from build123d import *

# Parameters (mm, degrees)
F0_W      = 58
F0_H      = 54
F1_DEPTH  = 10
F3_DEPTH  = 10
F5_DEPTH  = 50
F4_R      = 6
F4_W      = 10
F4_H      = 44
F7_DEPTH  = 50
F9_DEPTH  = 62.001
F10_DEPTH = 60.001
F11_DEPTH = 10.001


with BuildPart() as f1:
    # F0 (on Top) → F1 (new body)
    with BuildSketch(Plane.XY):
        Rectangle(F0_W, F0_H)
        Polygon((-29, -27), (-29, 27), (-81, 27), (-81, 7), align=None)
    extrude(amount=F1_DEPTH)

    # F2 (on face) → F3 (join)
    with BuildSketch(Plane(origin=(0, 27, 0), x_dir=(-1, 0, 0), z_dir=(0, 1, 0))):
        Polygon((19, 60), (-29, 10), (19, 10), align=None)
    extrude(amount=-F3_DEPTH)

    # F4 (on face) → F5 (join)
    with BuildSketch(Plane.XY.offset(10)):
        Polygon((-81, 27), (-81, 17), (-29, 17), (-19, 17), (-19, 27), align=None)
    extrude(amount=F5_DEPTH)

    # F4 (on face) → F7 (join)
    with BuildSketch(Plane.XY.offset(10)):
        with Locations((17, -5)):
            Circle(F4_R)
        with Locations((-5, -5)):
            Circle(F4_R)
        with Locations((-24, -5)):
            Rectangle(F4_W, F4_H)
    extrude(amount=F7_DEPTH)

    # F8 (on face) → F9 (cut, through all)
    with BuildSketch(Plane.YZ.offset(-19)):
        Polygon((-27, 60), (-27, 10), (17, 60), align=None)
    extrude(amount=-F9_DEPTH, mode=Mode.SUBTRACT)

    # F10 (cut, through all): faces of the model
    f10_faces = [f1.faces().sort_by_distance(p)[0] for p in [
        (-5, -5, 60),
        (17, -5, 60),
    ]]
    extrude(f10_faces, amount=-F10_DEPTH, mode=Mode.SUBTRACT)

    # F6 (on face) → F11 (cut, through all)
    with BuildSketch(Plane.XZ.offset(-17)):
        with BuildLine():
            ThreePointArc((-56.470110421, 44), (-59.8754155453, 47.4053051244), (-63.2807206697, 44))
            Line((-63.2807206697, 44), (-63.2807206697, 24))
            ThreePointArc((-63.2807206697, 24), (-59.8754155453, 20.5946948756), (-56.470110421, 24))
            Line((-56.470110421, 24), (-56.470110421, 44))
        make_face()
        with BuildLine():
            ThreePointArc((-34.5057800598, 44), (-37.8754155453, 47.3696354855), (-41.2450510308, 44))
            Line((-41.2450510308, 44), (-41.2450510308, 24))
            ThreePointArc((-41.2450510308, 24), (-37.8754155453, 20.6303645145), (-34.5057800598, 24))
            Line((-34.5057800598, 24), (-34.5057800598, 44))
        make_face()
    extrude(amount=-F11_DEPTH, mode=Mode.SUBTRACT)


solid = f1.part
Could you check a few things on this model? Use its own coordinates, in mm. A direction names the side the tool comes from. Round coordinates to 2 decimals unless told otherwise and drop trailing zeros. Loops run counter-clockwise (first coordinate to the right, second up) from the corner with the lowest first, then second, coordinate; pieces in that order, holes last. Notation, with made-up numbers: (7, -24.75) - (54, -24.75) arc R9 ccw to (54, -16.75) - close; hole circle Ø7 at (69.25, 68). An arc over 180 degrees is marked (long way). Write item = value, one per line.
1) I need wall thicknesses on line 1 along Z through (x, y) = (5, -7); line 2 along X through (y, z) = (9.5, 21.5); line 3 along Y through (x, z) = (-51.5, 37.5). Which ranges of each line are inside material? Lowest first, please. Write a range as from..to.
Computed:
line_1 = 0..10
line_2 = -29..-19
line_3 = 17..27
2) Imagine slicing it at C-C (z = 55). Please give me the cut outline in (x, y).
Computed:
outline = (-81, 17) - (-29, 17) - (-29, 12.6) - (-19, 12.6) - (-19, 17) - (-14.2, 17) - (-14.2, 27) - (-81, 27) - close
3) Imagine slicing it at D-D (y = 19). Please give me the cut outline in (x, z).
Computed:
outline = (-81, 0) - (29, 0) - (29, 10) - (-19, 60) - (-81, 60) - close; hole (-63.28, 24) arc R3.41 ccw to (-56.47, 24) - (-56.47, 44) arc R3.41 ccw to (-63.28, 44) - close; hole (-41.25, 24) arc R3.37 ccw to (-34.51, 24) - (-34.51, 44) arc R3.37 ccw to (-41.25, 44) - close
4) If we mould it in two halves opening along Z, with no side actions, what happens to faces 6 (the flat face through (-24, -5, 35)), 7 (the cylindrical face through (-59.95, 21.93, 20.596)), 8 (the flat face through (-55, 17, 35))? For each: pulls with the +Z half, pulls with the -Z half, needs draft (parallel to the pull), parting line crosses it, or undercut.
Computed:
face_6 = pulls with the +Z half
face_7 = undercut
face_8 = needs draft
5) Imagine slicing it at A-A (x = 17). Please give me the cut outline in (y, z), and give its area (3 significant figures).
Computed:
outline = (-27, 0) - (-11, 0) - (-11, 10) - (-27, 10) - close; (1, 0) - (27, 0) - (27, 22.5) - (17, 22.5) - (17, 10) - (1, 10) - close
area = 545 mm2
6) On a 3-axis mill with a long thin cutter (end or side, diameter ignored), from which of +Z, -Z, +X, -X, +Y, -Y can I reach the whole of each face in a straight line? I mean faces 1 (the flat face through (0, -27, 5)), 2 (the flat face through (-19, 4, 24)), 3 (the flat face through (-50, 22, 60)), 4 (the flat face through (-50, 0, 10)), 5 (the flat face through (-34.506, 22, 34)). Say none if no direction works.
Computed:
face_1 = +Z, -Z, +X, -X, -Y
face_2 = +Z, +X, -Y
face_3 = +Z, +X, -X, +Y, -Y
face_4 = +Z, -X, -Y
face_5 = +Y, -Y
7) Imagine slicing it at B-B (z = 36). Please give me the cut outline in (x, y), and give its area (3 significant figures).
Computed:
outline = (-81, 17) - (-63.28, 17) - (-63.28, 27) - (-81, 27) - close; (-56.47, 17) - (-41.25, 17) - (-41.25, 27) - (-56.47, 27) - close; (-34.51, 17) - (-29, 17) - (-29, -4.12) - (-19, -4.12) - (-19, 17) - (4.04, 17) - (4.04, 27) - (-34.51, 27) - close
area = 926 mm2
8) I'm going to push flat-ended pins straight in: P1, Ø1.5, axis at x = -23.5, z = 45, coming from the -Y side; P2, Ø14, axis at x = -5, y = -5, coming from the +Z side; P3, Ø5, axis at y = 22.5, z = 36, coming from the +X side. Where does each tip first touch, or does it pass through?
Computed:
P1 = 3.14
P2 = 10
P3 = 6.44
